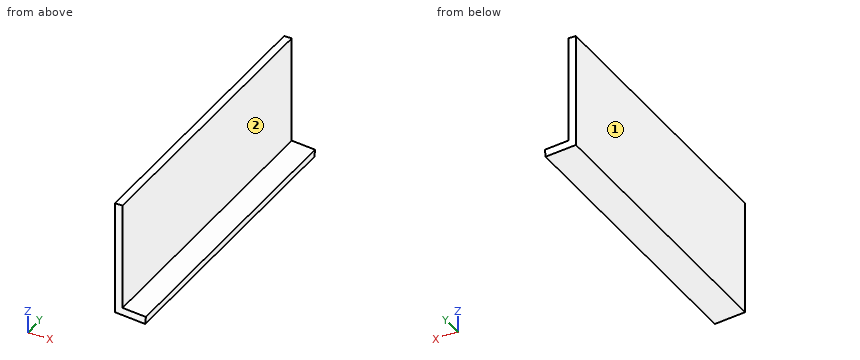
from build123d import *

# Parameters (mm, degrees)
F0_W     = 1016
F0_H     = 381
F1_DEPTH = 25.4
F3_DEPTH = 1016


with BuildPart() as f1:
    # F0 (on Right) → F1 (new body)
    with BuildSketch(Plane.YZ):
        Rectangle(F0_W, F0_H)
    extrude(amount=F1_DEPTH)

    # F2 (on face) → F3 (join, through all)
    with BuildSketch(Plane.XZ.offset(508)):
        Polygon((0, -165.002976), (0, -190.5), (101.213381, -199.355023), (103.427137, -174.051678), align=None)
    extrude(amount=-F3_DEPTH)


solid = f1.part
Work out the finished part from the listing and answer in its coordinate system (mm). Face numbers are marked on the shaded views. A direction names the side the tool comes from. Round coordinates to 2 decimals unless told otherwise and drop trailing zeros. Loops run counter-clockwise (first coordinate to the right, second up) from the corner with the lowest first, then second, coordinate; pieces in that order, holes last. Notation, with made-up numbers: (75, 74) -> (94, 74) arc R12 cw to (94, 81) -> close; hole circle Ø9 at (49.25, -17.5). An arc over 180 degrees is marked (long way). Use one line per item in the form item = value.
(1) Find section C-C on x = 92. Give the vertices of the cut face in (y, z).
Answer list:
outline = (-508, -198.55) -> (508, -198.55) -> (508, -173.05) -> (-508, -173.05) -> close
(2) Straight lines are drawn through the part: line 1 (X direction, y = -354, z = 36); line 2 (Z direction, x = 12.5, y = 177.5); line 3 (Z direction, x = 71, y = 40). For each, find the intervals that lie inside material, in ascending order.
Answer list:
line_1 = 0 to 25.4
line_2 = -191.59 to 190.5
line_3 = -196.71 to -171.21
(3) A tool of negligible diameter and unlimited length cuts with its end or side. For the marked faces 1 and 2, from which of +Z, -Z, +X, -X, +Y, -Y can it reach the whole face along a straight path? Write none if from no direction.
Answer list:
face_1 = +Z, -Z, -X, +Y, -Y
face_2 = +Z, +X, +Y, -Y
(4) Flat-ended cylindrical pins translate along their axes: P1, Ø3, axis at x = 89.5, y = 219, coming from the -Z side; P2, Ø12, axis at x = 90, y = -347.5, coming from the -Z side; P3, Ø10, axis at x = 67, y = 359, coming from the +Z side. Find the tip coordinate at first contact, or state that the pin passes through.
Answer list:
P1 = -198.46
P2 = -198.9
P3 = -170.43
(5) Find section B-B on z = -11. Give the vertices of the cut face in (x, y).
Answer list:
outline = (0, -508) -> (25.4, -508) -> (25.4, 508) -> (0, 508) -> close
(6) Find section A-A on y = 208.5. Give the vertices of the cut face in (x, z), then the cut area to 3 significant figures.
Answer list:
outline = (0, -190.5) -> (101.21, -199.36) -> (103.43, -174.05) -> (25.4, -167.23) -> (25.4, 190.5) -> (0, 190.5) -> close
area = 11,700 mm2
